Geometry: final body of the model. Coordinates: model frame, mm. A direction names the side the tool comes from. Coordinates: 2 decimals unless noted, no trailing zeros. Loops run counter-clockwise (first coordinate to the right, second up) from the corner with the lowest first, then second, coordinate; pieces in that order, holes last. Notation, with made-up numbers: (1.25, 29.5) - (27.25, 29.5) arc R13 ccw to (27.25, 42.5) - close; hole circle Ø1 at (46.25, 7.5). An arc over 180 degrees is marked (long way). Return JSON: item names as keys, results as strings.
from build123d import *

# Parameters (mm, degrees)
EXTRUDE_1_DEPTH          = 2
SKETCH_2_R               = 1.6
SKETCH_2_R_2             = 2.1
CUT_EXTRUDE_1_DEPTH      = 63.985380966
CUT_EXTRUDE_4_DEPTH      = 63.89004862
CUT_EXTRUDE_4_DEPTH_BACK = 63.89004862
CHAMFER_1_SIZE           = 1


with BuildPart() as part:
    # 草图1 → 凸台-拉伸1 (new, symmetric)
    with BuildSketch(Plane(origin=(0, 0, 0), x_dir=(1, 0, 0), z_dir=(0, 1, 0))):
        with BuildLine():
            Line((-18.511332271, 2.604722665), (-9.84807753, 51.736481777))
            ThreePointArc((-9.84807753, 51.736481777), (0, 60), (9.84807753, 51.736481777))
            Line((9.84807753, 51.736481777), (18.511332271, 2.604722665))
            ThreePointArc((18.511332271, 2.604722665), (18.739215976, 0), (18.511332271, -2.604722665))
            Line((18.511332271, -2.604722665), (9.84807753, -51.736481777))
            ThreePointArc((9.84807753, -51.736481777), (0, -60), (-9.84807753, -51.736481777))
            Line((-9.84807753, -51.736481777), (-18.511332271, -2.604722665))
            ThreePointArc((-18.511332271, -2.604722665), (-18.739215976, 0), (-18.511332271, 2.604722665))
        make_face()
    extrude(amount=EXTRUDE_1_DEPTH, both=True)

    # 草图2 → 切除-拉伸1 (cut, through all)
    with BuildSketch(Plane(origin=(0, 2, 0), x_dir=(1, 0, 0), z_dir=(0, 1, 0))):
        with Locations(Location((0, 50, 0), (0, 0, 270))):
            Circle(SKETCH_2_R)
        with Locations(Location((0, -50, 0), (0, 0, 270))):
            Circle(SKETCH_2_R_2)
    extrude(amount=-CUT_EXTRUDE_1_DEPTH, mode=Mode.SUBTRACT)

    # 草图6 → 切除-拉伸4 (cut, two sides: drawn at the far end of the back side and taken through both)
    with BuildSketch(Plane(origin=(0, 0, 0), x_dir=(1, 0, 0), z_dir=(0, 1, 0)).offset(-CUT_EXTRUDE_4_DEPTH_BACK)):
        with BuildLine():
            Line((-1.969615506, 38.829755389), (-8.663254741, 0.868240888))
            ThreePointArc((-8.663254741, 0.868240888), (-8.739215976, 0), (-8.663254741, -0.868240888))
            Line((-8.663254741, -0.868240888), (-1.969615506, -38.829755389))
            ThreePointArc((-1.969615506, -38.829755389), (0, -40.482459034), (1.969615506, -38.829755389))
            Line((1.969615506, -38.829755389), (8.663254741, -0.868240888))
            ThreePointArc((8.663254741, -0.868240888), (8.739215976, 0), (8.663254741, 0.868240888))
            Line((8.663254741, 0.868240888), (1.969615506, 38.829755389))
            ThreePointArc((1.969615506, 38.829755389), (0, 40.482459034), (-1.969615506, 38.829755389))
        make_face()
    extrude(amount=CUT_EXTRUDE_4_DEPTH + CUT_EXTRUDE_4_DEPTH_BACK, mode=Mode.SUBTRACT)

    # 倒角1
    chamfer_1_edges = [part.edges().sort_by_distance(p)[0] for p in [
        (-14.179704901, -2, 27.170602221),
        (-18.739215976, -2, 0),
        (-14.179704901, -2, -27.170602221),
        (0, -2, -60),
        (-18.739215976, 2, 0),
        (-14.179704901, 2, 27.170602221),
        (0, 2, 60),
        (14.179704901, 2, 27.170602221),
        (18.739215976, 2, 0),
        (14.179704901, 2, -27.170602221),
        (0, -2, 40.482459034),
        (-5.316435124, -2, 19.848998139),
        (-8.739215976, -2, 0),
        (-5.316435124, -2, -19.848998139),
        (0, -2, -40.482459034),
        (5.316435124, -2, -19.848998139),
        (8.739215976, -2, 0),
        (5.316435124, -2, 19.848998139),
        (0, 2, 40.482459034),
        (5.316435124, 2, 19.848998139),
        (8.739215976, 2, 0),
        (5.316435124, 2, -19.848998139),
        (0, 2, -40.482459034),
        (-5.316435124, 2, -19.848998139),
        (-8.739215976, 2, 0),
        (-5.316435124, 2, 19.848998139),
        (0, 2, -60),
        (14.179704901, -2, -27.170602221),
        (-14.179704901, 2, -27.170602221),
        (18.739215976, -2, 0),
        (14.179704901, -2, 27.170602221),
        (0, -2, 60),
    ]]
    chamfer(chamfer_1_edges, length=CHAMFER_1_SIZE)


solid = part.part
Item 1: Section query D-D, the plane z = 50. Return loops of the section in (x, y), and give its area (3 significant figures).
Worked out:
{"outline": "(-10.15, -1) - (-9.14, -2) - (-2.1, -2) - (-2.1, 2) - (-9.14, 2) - (-10.15, 1) - close; (2.1, -2) - (9.14, -2) - (10.15, -1) - (10.15, 1) - (9.14, 2) - (2.1, 2) - close", "area": "62.4 mm^2"}
Item 2: Reachability of faces 1 (the face through (-14.12, 0.01, 27.51)), 2 (the face through (-5.849, -1.493, -19.669)), 3 (the face through (5.27, -0.01, 20.11)), 4 (the face through (5.755, 1.493, -20.2)), 5 (the face through (14.12, 0.01, -27.51)) from +Z, -Z, +X, -X, +Y, -Y: full face, straight path, thin tool, end or side. Return the list, or none.
Worked out:
{"face 1": "+Z, -X, +Y, -Y", "face 2": "-Y", "face 3": "+Y, -Y", "face 4": "+Y", "face 5": "-Z, +X, +Y, -Y"}
Item 3: Ray query, probe 1 along X at (y, z) = (0.45, 23); probe 2 along Z at (x, y) = (0.5, -1.5); probe 3 along X at (y, z) = (0.25, -50). Return the intervals inside material, ascending. Write a range as from..to.
Worked out:
{"probe 1": "-14.92..-4.76, 4.76..14.92", "probe 2": "-59.49..-51.52, -48.48..-40.93, 40.93..47.96, 52.04..59.49", "probe 3": "-10.15..-1.6, 1.6..10.15"}
Item 4: Section query C-C, the plane y = -0.1. Return loops of the section in (x, z).
Worked out:
{"outline": "(-18.51, -2.6) - (-9.85, -51.74) arc R10 ccw to (9.85, -51.74) - (18.51, -2.6) arc R15 ccw to (18.51, 2.6) - (9.85, 51.74) arc R10 ccw to (-9.85, 51.74) - (-18.51, 2.6) arc R15 ccw to start; hole (-8.66, -0.87) - (-1.97, -38.83) arc R2 ccw to (1.97, -38.83) - (8.66, -0.87) arc R5 ccw to (8.66, 0.87) - (1.97, 38.83) arc R2 ccw to (-1.97, 38.83) - (-8.66, 0.87) arc R5 ccw to start; hole circle Ø4.2 at (0, 50); hole circle Ø3.2 at (0, -50)"}
Item 5: First-contact query: pin 1 Ø4 at (x, z) = (0, -50) entering from +Y; pin 2 Ø3.5 at (x, z) = (0, 50) entering from +Y; pin 3 Ø1.5 at (x, y) = (2.5, 1) entering from +Z; pin 4 Ø1.5 at (x, y) = (-8, 0) entering from +Z. Flat tips, straight axial feed; report the tip coordinate or a pass-through.
Worked out:
{"pin 1": "y = 2", "pin 2": "through", "pin 3": "z = 59.85", "pin 4": "z = 56.89"}
Item 6: Section query B-B, the plane x = 0. Return loops of the section in (y, z).
Worked out:
{"outline": "(-2, -59) - (-1, -60) - (1, -60) - (2, -59) - (2, -51.6) - (-2, -51.6) - close; (-2, -48.4) - (2, -48.4) - (2, -41.48) - (1, -40.48) - (-1, -40.48) - (-2, -41.48) - close; (-2, 41.48) - (-1, 40.48) - (1, 40.48) - (2, 41.48) - (2, 47.9) - (-2, 47.9) - close; (-2, 52.1) - (2, 52.1) - (2, 59) - (1, 60) - (-1, 60) - (-2, 59) - close"}
Item 7: Mould query, pull axis X, two halves, no side actions, for faces 6 (the face through (-13.74, 1.51, -26.74)), 7 (the face through (0.2, 1.8, 59.2)), 8 (the face through (5.849, 1.493, 19.669)). Classes: +X half, -X half, draft (parallel to the pull), parting line (faces both ways), or undercut.
Worked out:
{"face 6": "-X half", "face 7": "parting line", "face 8": "undercut"}
Item 8: Section query A-A, the plane z = -6.5. Return loops of the section in (x, y).
Worked out:
{"outline": "(-17.82, -1) - (-16.81, -2) - (-8.69, -2) - (-7.67, -1) - (-7.67, 1) - (-8.69, 2) - (-16.81, 2) - (-17.82, 1) - close; (7.67, -1) - (8.69, -2) - (16.81, -2) - (17.82, -1) - (17.82, 1) - (16.81, 2) - (8.69, 2) - (7.67, 1) - close"}
